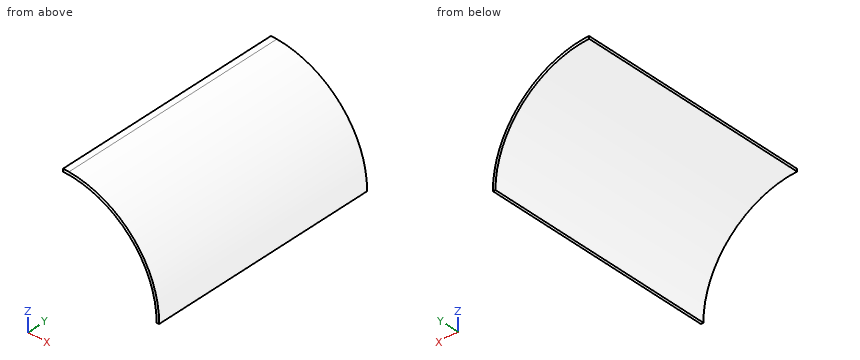
from build123d import *

# Parameters (mm, degrees)
F0_W     = 290
F0_H     = 290
F1_DEPTH = 700
F3_DEPTH = 795
F5_DEPTH = 770


with BuildPart() as f1:
    # F0 (on Front) → F1 (new body)
    with BuildSketch(Plane.XZ):
        with Locations((145, 145)):
            Rectangle(F0_W, F0_H)
    extrude(amount=F1_DEPTH)

    # F2 (on face) → F3 (cut)
    with BuildSketch(Plane.XZ):
        with BuildLine():
            ThreePointArc((18.21568, 290), (211.733128, 199.092972), (289.675921, 0))
            Line((289.675921, 0), (290, 0))
            Line((290, 0), (290, 290))
            Line((290, 290), (18.21568, 290))
        make_face()
    extrude(amount=F3_DEPTH, mode=Mode.SUBTRACT)

    # F4 (on face) → F5 (cut)
    with BuildSketch(Plane.XZ.offset(700)):
        with BuildLine():
            Line((0, 0), (282.123595, 0))
            ThreePointArc((282.123595, 0), (199.483979, 199.530675), (0, 282.282948))
            Line((0, 282.282948), (0, 0))
        make_face()
    extrude(amount=-F5_DEPTH, mode=Mode.SUBTRACT)


solid = f1.part
The listing builds one solid part. Answer for the finished solid, in the listing's coordinates (mm). Coordinates: 2 decimals unless noted, no trailing zeros. Loops run counter-clockwise (first coordinate to the right, second up) from the corner with the lowest first, then second, coordinate; pieces in that order, holes last.
1) Find section B-B on x = 194. Write down the section's boundary in (y, z).
2) Flat-ended cylindrical pins translate along their axes: pin 1 Ø10 at (x, y) = (254, -591) entering from +Z; pin 2 Ø2 at (x, y) = (173, -185.5) entering from +Z; pin 3 Ø1 at (x, y) = (196.5, -563) entering from +Z. Find the tip coordinate at first contact, or state that the pin passes through.
3) Find section C-C on z = 31. Write down the section's boundary in (x, y).
4) Find the intervals of material crossed by L1, parallel to X at y = -72, z = 216; L2, parallel to Z at x = 203.5, y = -577; L3, parallel to X at y = -150, z = 143, in increasing order.
5) Find section A-A on y = -376. Write down the section's boundary in (x, z).
Values:
1. outline: (-700, 204.87) - (0, 204.87) - (0, 216.47) - (-700, 216.47) - close
2. pin 1: stops at z = 149.54
2. pin 2: stops at z = 234.38
2. pin 3: stops at z = 214.66
3. outline: (280.41, -700) - (288.2, -700) - (288.2, 0) - (280.41, 0) - close
4. L1: x = 181.54 to 194.53
4. L2: z = 195.43 to 207.54
4. L3: x = 243.2 to 252.78
5. outline: (0, 282.28) arc R282.34 cw to (282.12, 0) - (289.68, 0) arc R288.76 ccw to (18.22, 290) - (0, 290) - close
